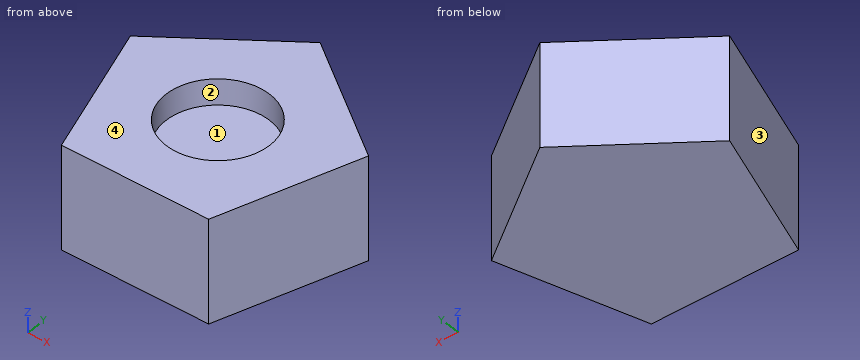
```python
from build123d import *

# Parameters (mm, degrees)
F1_DEPTH = 15
F2_R     = 10
F3_DEPTH = 5


with BuildPart() as f1:
    # F0 (on Top) → F1 (new body)
    with BuildSketch(Plane.XY):
        Polygon((0, -19.677398), (0, 24.322602), (-23.132169, 7.516097), (-14.296467, -19.677398), align=None)
        Polygon((23.132169, 7.516097), (0, 24.322602), (0, -19.677398), (14.296467, -19.677398), align=None)
    extrude(amount=F1_DEPTH)

    # F2 (on face) → F3 (join)
    with BuildSketch(Plane.XY.offset(15)):
        Polygon((0, 24.322602), (-23.132169, 7.516097), (-14.296467, -19.677398), (14.296467, -19.677398), (23.132169, 7.516097), align=None)
        Circle(F2_R, mode=Mode.SUBTRACT)
    extrude(amount=F3_DEPTH)


solid = f1.part
```
Verification items for the finished model (mm, model axes). Face numbers are marked on the shaded views. Give positions to 0.01 mm unless a question says otherwise; leave off trailing zeros. Order: outer loops, then holes, each group sorted by start corner. A loop starts at its lowest first (then second) coordinate and runs counter-clockwise, first axis right, second up. Notation, with made-up numbers: (-6, 0) -> (24, 0) arc R32 ccw to (24, 35) -> close; hole circle Ø3 at (59, 61). An arc over 180 degrees is marked (long way). Use a Markdown table: item, result.
1) Material ranges on probe 1 along Y at (x, z) = (0, 18.4); probe 2 along Y at (x, z) = (-7, 16.75); probe 3 along Z at (x, y) = (-1, -0.5), recorded low to high.
Results:
| item | result |
|---|---|
| probe 1 | -19.68 to -10, 10 to 24.32 |
| probe 2 | -19.68 to -7.14, 7.14 to 19.24 |
| probe 3 | 0 to 15 |
2) Depth check by flat-ended pin: pin 1 Ø6 at (x, y) = (1.5, -4) entering from +Z; pin 2 Ø1 at (x, z) = (8.5, 13.5) entering from +Y; pin 3 Ø1.5 at (y, z) = (-10.5, 2) entering from +X. Enter the tip coordinate at first touch or a pass-through.
Results:
| item | result |
|---|---|
| pin 1 | z = 15 |
| pin 2 | y = 18.51 |
| pin 3 | x = 17.52 |
3) Section check A-A, the plane z = 18. Record the boundary of the cut face in (x, y), then the cut area to 3 significant figures.
Results:
| item | result |
|---|---|
| outline | (-23.13, 7.52) -> (-14.3, -19.68) -> (14.3, -19.68) -> (23.13, 7.52) -> (0, 24.32) -> close; hole circle Ø20 at (0, 0) |
| area | 1,090 mm² |
4) Section check C-C, the plane y = -7. Record the boundary of the cut face in (x, z).
Results:
| item | result |
|---|---|
| outline | (-18.42, 0) -> (18.42, 0) -> (18.42, 20) -> (7.14, 20) -> (7.14, 15) -> (-7.14, 15) -> (-7.14, 20) -> (-18.42, 20) -> close |
5) Mould release check, pull along Y, two halves, no side actions. Record for the marked faces 1, 2, 3 and 4: pulls with the +Y half, pulls with the -Y half, needs draft (parallel to the pull), parting line crosses it, or undercut.
Results:
| item | result |
|---|---|
| face 1 | undercut |
| face 2 | undercut |
| face 3 | pulls with the -Y half |
| face 4 | needs draft |
6) Section check D-D, the plane x = 5. Record the boundary of the cut face in (y, z).
Results:
| item | result |
|---|---|
| outline | (-19.68, 0) -> (20.69, 0) -> (20.69, 20) -> (8.66, 20) -> (8.66, 15) -> (-8.66, 15) -> (-8.66, 20) -> (-19.68, 20) -> close |
7) Section check B-B, the plane z = 2.25. Record the boundary of the cut face in (x, y).
Results:
| item | result |
|---|---|
| outline | (-23.13, 7.52) -> (-14.3, -19.68) -> (14.3, -19.68) -> (23.13, 7.52) -> (0, 24.32) -> close |
